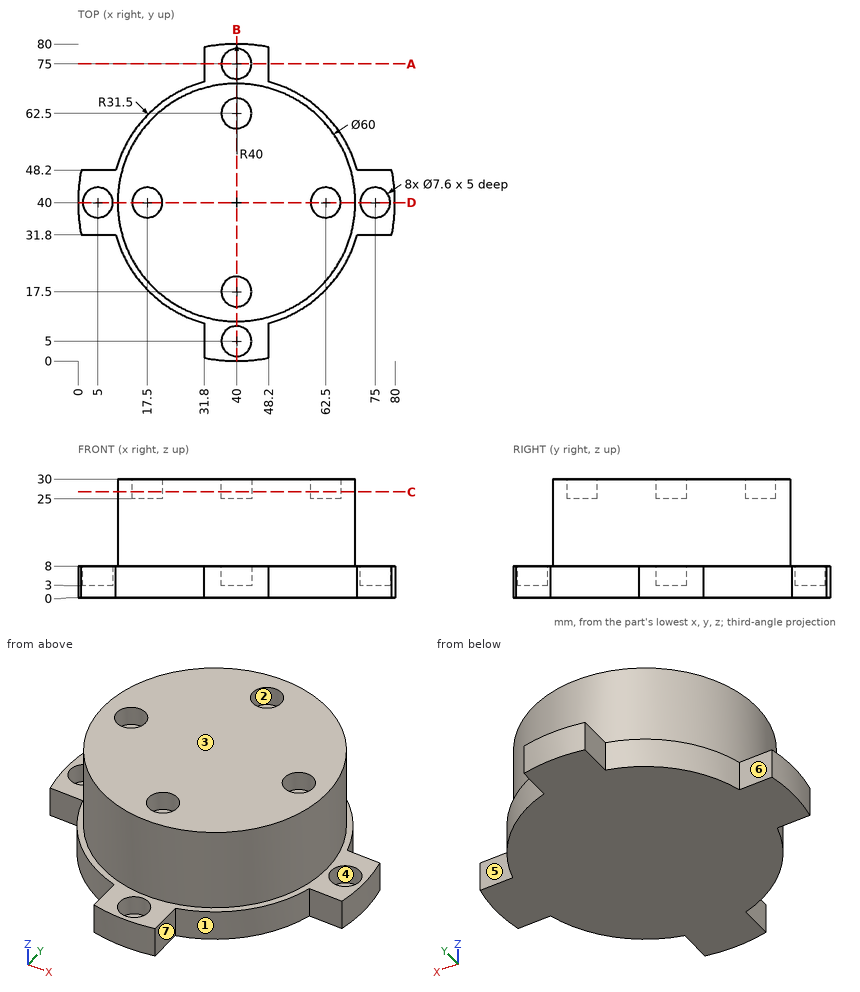
Part print with two shaded views. Sizes in mm from the minimum x, y, z corner. A direction names the side the tool comes from. Round coordinates to 2 decimals unless told otherwise and drop trailing zeros. Write each loop counter-clockwise with the first axis right and the second up, starting at its lowest first coordinate (ties: lowest second). Pieces come first, ordered by that corner, then holes. Notation, with made-up numbers: M -1.75,62.5 L 30.25,62.5 A27 cw 30.25,100.5 Z; hole C -35,-27 d7. An arc over 180 degrees is marked long. Use CSV: the item, a comma, the result in double quotes.
1. Wall check: probe 1 along Y at (x, z) = (40, 4.7); probe 2 along Y at (x, z) = (37.5, 7); probe 3 along X at (y, z) = (9, 5). Give the ranges that are in metal, low to high. Write a range as from..to.
Reply:
probe 1,"y = 0..1.2, 8.8..71.2, 78.8..80"
probe 2,"y = 0.08..2.14, 7.86..72.14, 77.86..79.92"
probe 3,"x = 31.8..48.2"
2. Saw through at B-B (x = 40). Give the cut face in (y, z).
Reply:
outline,"M 0,0 L 80,0 L 80,8 L 78.8,8 L 78.8,3 L 71.2,3 L 71.2,8 L 70,8 L 70,30 L 66.3,30 L 66.3,25 L 58.7,25 L 58.7,30 L 21.3,30 L 21.3,25 L 13.7,25 L 13.7,30 L 10,30 L 10,8 L 8.8,8 L 8.8,3 L 1.2,3 L 1.2,8 L 0,8 Z"
3. Saw through at A-A (y = 75). Give the cut face in (x, z), plus the area to 3 significant figures.
Reply:
outline,"M 31.8,0 L 48.2,0 L 48.2,8 L 43.8,8 L 43.8,3 L 36.2,3 L 36.2,8 L 31.8,8 Z"
area,"93.2 mm²"
4. Flat gauge pins, fed straight in: pin 1 (2.5 mm diameter, centred on y = 6, z = 2, fed in from +X); pin 2 (6 mm diameter, centred on x = 40, y = 75, fed in from +Z); pin 3 (6.5 mm diameter, centred on y = 6, z = 4.5, fed in from -X). Where does each tip first touch, or does it go through?
Reply:
pin 1,"stops at x = 48.2"
pin 2,"stops at z = 3"
pin 3,"stops at x = 31.8"
5. Tool access for the marked faces 4, 5, 6 and 7: list every direction of +Z, -Z, +X, -X, +Y, -Y with a clear straight run to the whole face (end or side of a thin tool).
Reply:
face 4,"+Z"
face 5,"+Z, -Z, +X, +Y"
face 6,"+Z, -Z, -X, +Y"
face 7,"+Z, -Z, +X, -Y"
6. Two-plate mould, pull along Y, no slides. Class the marked faces 1, 2 and 3: +Y half, -Y half, draft (parallel to the pull), parting line (faces both ways), or undercut.
Reply:
face 1,"-Y half"
face 2,"undercut"
face 3,"draft"
7. Saw through at C-C (z = 26.75). Give the cut face in (x, y).
Reply:
outline,"C 40,40 d60; hole C 17.5,40 d7.6; hole C 40,17.5 d7.6; hole C 40,62.5 d7.6; hole C 62.5,40 d7.6"
